```python
from build123d import *

# Parameters (mm, degrees)
F0_W      = 20
F0_H      = 37.5
F1_DEPTH  = 5
F3_D      = 3
F4_W      = 6.5
F4_H      = 24
F5_DEPTH  = 6
F6_R      = 2
F10_DEPTH = 50
F14_W     = 23.2
F14_H     = 31
F15_DEPTH = 6
F16_W     = 20.2
F16_H     = 30.2
F17_DEPTH = 3.5
F19_DEPTH = 14
F20_W     = 10
F20_H     = 5
F21_DEPTH = 4
F22_W     = 11
F22_H     = 2
F23_DEPTH = 3
F24_W     = 11
F24_H     = 4
F25_DEPTH = 3
F27_DEPTH = 2
F29_DEPTH = 2
F30_R     = 0.4
F31_DEPTH = 70


# Not quite as in the source:
# - a feature names something its author has since deleted; it is built from what else it names


with BuildPart() as f1:
    # F0 (on Top) → F1 (new body)
    with BuildSketch(Plane.XY):
        Rectangle(F0_W, F0_H)
    extrude(amount=F1_DEPTH)

    # F3 (through all)
    with Locations(Plane(origin=(0, 0, 0), x_dir=(1, 0, 0), z_dir=(0, 0, -1))):
        with Locations((-6.75, 15), (-6.75, -15)):
            Hole(F3_D / 2)

    # F4 (on Top) → F5 (cut)
    with BuildSketch(Plane.XY):
        with Locations((-6.75, 0)):
            Rectangle(F4_W, F4_H)
    extrude(amount=F5_DEPTH, mode=Mode.SUBTRACT)

    # F6
    f6_edges = [f1.edges().sort_by_distance(p)[0] for p in [
        (-10, -18.75, 2.5),
        (10, -18.75, 2.5),
        (10, 18.75, 2.5),
        (-10, 18.75, 2.5),
        (-10, -12, 2.5),
        (-10, 12, 2.5),
    ]]
    fillet(f6_edges, radius=F6_R)

    # F9 (on line) → F10 (cut)
    with BuildSketch(Plane(origin=(5.0561841595, -5.0561841595, 0), x_dir=(0.7071067812, 0.7071067812, 0), z_dir=(0.7071067812, -0.7071067812, 0))):
        with BuildLine():
            ThreePointArc((10.5836309448, 0.525), (11.626613447, 0.9570174977), (12.0586309448, 2))
            ThreePointArc((12.0586309448, 2), (9.5406484425, 3.0429825023), (10.5836309448, 0.525))
        make_face()
    extrude(amount=-F10_DEPTH, mode=Mode.SUBTRACT)

    # F11: F1 across plane


with BuildPart() as f1_1:
    add(f1.part)
    add(f1.part.mirror(Plane.XZ), mode=Mode.INTERSECT)

    # F14 (on line) → F15 (join)
    with BuildSketch(Plane(origin=(2.3153133603, 0, 1.9427785867), x_dir=(0, 1, 0), z_dir=(0.7660444431, 0, 0.6427876097))):
        with Locations((0, 19.490919118)):
            Rectangle(F14_W, F14_H)
    extrude(amount=F15_DEPTH)

    # F16 (on face) → F17 (cut)
    with BuildSketch(Plane(origin=(6.911580019, 0, 5.7995042448), x_dir=(0, 1, 0), z_dir=(0.7660444431, 0, 0.6427876097))):
        with Locations((0, 18.390919118)):
            Rectangle(F16_W, F16_H)
    extrude(amount=-F17_DEPTH, mode=Mode.SUBTRACT)

    # F18 (on Front) → F19 (join, symmetric)
    with BuildSketch(Plane.XZ):
        Polygon((4.3462666587, 8.8567256581), (-0.25, 5), (7.582443736, 5), align=None)
    extrude(amount=F19_DEPTH, both=True)

    # F20 (on face) → F21 (cut)
    with BuildSketch(Plane(origin=(4.2304244681, 0, 3.5497476109), x_dir=(0, 1, 0), z_dir=(0.7660444431, 0, 0.6427876097))):
        with Locations((0, 6.490919118)):
            Rectangle(F20_W, F20_H)
    extrude(amount=-F21_DEPTH, mode=Mode.SUBTRACT)

    # F22 (on face) → F23 (cut)
    with BuildSketch(Plane(origin=(6.911580019, 0, 5.7995042448), x_dir=(0, 1, 0), z_dir=(0.7660444431, 0, 0.6427876097))):
        with Locations((4.6, 34.490919118)):
            Rectangle(F22_W, F22_H)
    extrude(amount=-F23_DEPTH, mode=Mode.SUBTRACT)

    # F24 (on face) → F25 (cut)
    with BuildSketch(Plane(origin=(6.911580019, 0, 5.7995042448), x_dir=(0, 1, 0), z_dir=(0.7660444431, 0, 0.6427876097))):
        with Locations((-4.6, 1.990919118)):
            Rectangle(F24_W, F24_H)
    extrude(amount=-F25_DEPTH, mode=Mode.SUBTRACT)

    # F26 (on face) → F27 (join)
    with BuildSketch(Plane.XZ.offset(11.6)):
        Polygon((-15.5801492416, 32.6041033948), (-20.1764159003, 28.7473777367), (-18.2480530712, 26.4492444073), (-13.6517864125, 30.3059700655), align=None)
    extrude(amount=F27_DEPTH)

    # F28 (on face) → F29 (join)
    with BuildSketch(Plane(origin=(0, 11.6, 0), x_dir=(-1, 0, 0), z_dir=(0, 1, 0))):
        Polygon((20.1764159003, 28.7473777367), (15.5801492416, 32.6041033948), (13.6517864125, 30.3059700655), (18.2480530712, 26.4492444073), align=None)
    extrude(amount=F29_DEPTH)

    # F30 (on face) → F31 (cut)
    with BuildSketch(Plane.YZ.offset(10)):
        with Locations((0, 2.5)):
            Circle(F30_R)
    extrude(amount=-F31_DEPTH, mode=Mode.SUBTRACT)


solid = f1_1.part
```
Input: part model. Units: mm. Frame: model coordinates. A direction names the side the tool comes from. Coordinates: 2 decimals unless noted, no trailing zeros. Write each loop counter-clockwise with the first axis right and the second up, starting at its lowest first coordinate (ties: lowest second). Pieces come first, ordered by that corner, then holes.
1) Pin query (flat end, axial travel): pin 1 Ø1.5 at (x, z) = (-1.5, 6.5) entering from +Y; pin 2 Ø5 at (x, z) = (-15.5, 28.5) entering from -Y; pin 3 Ø12 at (y, z) = (-7, 28) entering from -X; pin 4 Ø2 at (y, z) = (15.5, 2) entering from -X. Return the tip coordinate at first contact, or that it passes through.
2) Section B-B on y = -15. State how many separate pieces and enclosed holes the cut face has, and give its area (3 significant figures).
3) Section C-C on z = 20.5. Output: boundary loops of the cut face in (x, y), and give its area (3 significant figures).
4) Section A-A on x = -6.75. Output: boundary loops of the cut face in (y, z), and give its area (3 significant figures).
5) Material intervals for line 1 along Y through (x, z) = (-8, 21); line 2 along Z through (x, y) = (3, 0); line 3 along X through (y, z) = (-15, 1), sorted ascending.
6) Set-up query: faces 1 (the flat face through (-16, -0.9, 31)), 2 (the flat face through (5.78, -4.68, 4.84)), 3 (the flat face through (-3.5, -0.2, 1.9)), 4 (the flat face through (4, -14, 6)), 5 (the flat face through (-1, -5, 8)). Return all of +Z, -Z, +X, -X, +Y, -Y with unobstructed straight access to the full face (end or side cutting, diameter ignored); none if empty.
7) Mould query, pull axis Y, two halves, no side actions, for faces 6 (the flat face through (-7, 11.6, 17)), 7 (the flat face through (0, -18.75, 2)), 8 (the flat face through (-1.3, 5, 4.6)), 9 (the flat face through (2, 0, 0)). Classes: pulls with the +Y half, pulls with the -Y half, needs draft (parallel to the pull), parting line crosses it, or undercut.
Check result:
1. pin 1: stops at y = 11.6
1. pin 2: stops at y = -13.6
1. pin 3: stops at x = -20.18
1. pin 4: stops at x = -10
2. separate pieces: 2
2. enclosed holes: 1
2. area: 75.3 mm2
3. outline: (-13.26, -11.6) - (-5.42, -11.6) - (-5.42, -10.1) - (-9.99, -10.1) - (-9.99, 10.1) - (-5.42, 10.1) - (-5.42, 11.6) - (-13.26, 11.6) - close
3. area: 89.4 mm2
4. outline: (-18.75, 0) - (-16.5, 0) - (-16.5, 5) - (-18.75, 5) - close; (-13.5, 0) - (-12, 0) - (-12, 5) - (-13.5, 5) - close; (-11.6, 12.75) - (11.6, 12.75) - (11.6, 22.08) - (10.1, 22.08) - (10.1, 16.64) - (-10.1, 16.64) - (-10.1, 22.08) - (-11.6, 22.08) - close; (12, 0) - (13.5, 0) - (13.5, 5) - (12, 5) - close; (16.5, 0) - (18.75, 0) - (18.75, 5) - (16.5, 5) - close
4. area: 144 mm2
5. line 1: y = -11.6 to -10.1, 10.1 to 11.6
5. line 2: z = 0 to 2.1, 2.9 to 5.79
5. line 3: x = -10 to -8.25, -5.25 to -1.57, 1.5 to 10
6. face 1: +Z, +X
6. face 2: +Z
6. face 3: -Z, -X
6. face 4: +Z, +X, -X, -Y
6. face 5: none
7. face 6: pulls with the +Y half
7. face 7: pulls with the -Y half
7. face 8: undercut
7. face 9: needs draft
